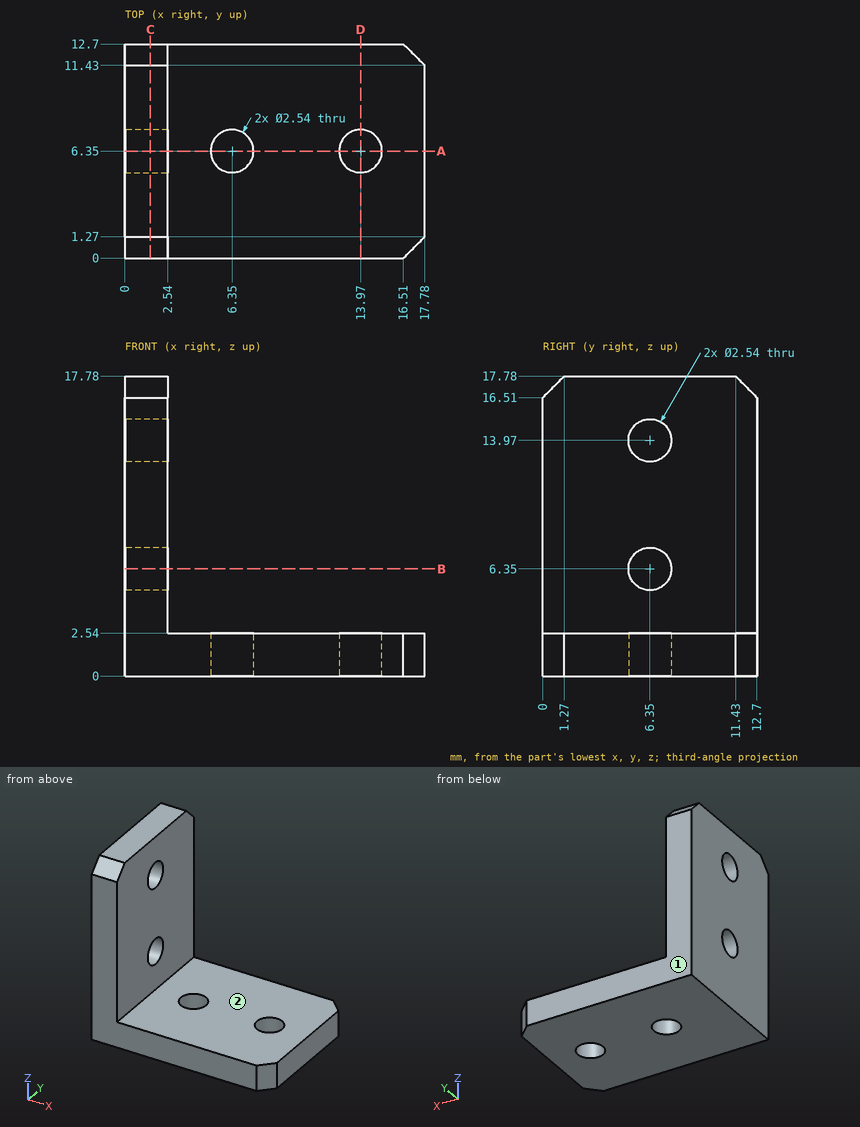
Source: three-view drawing plus pictorial views. Frame: mm from the lowest corner of the part. A direction names the side the tool comes from. Round coordinates to 2 decimals unless told otherwise and drop trailing zeros. Loops run counter-clockwise (first coordinate to the right, second up) from the corner with the lowest first, then second, coordinate; pieces in that order, holes last.
Q1. Section D-D, the plane x = 13.97. Return loops of the section in (y, z), plus the area to 3 significant figures.
Q2. Section A-A, the plane y = 6.35. Return loops of the section in (x, z), plus the area to 3 significant figures.
Q3. Section B-B, the plane z = 6.35. Return loops of the section in (x, y).
Q4. Ray query, line 1 (Y direction, x = 13.97, z = 1.9); line 2 (X direction, y = 11.5, z = 6.25). Return the intervals inside material, ascending.
Q5. Access query for the marked faces 1 and 2. Directions: +Z, -Z, +X, -X, +Y, -Y. A direction counts if a zero-diameter tool reaches every point of the face in a straight line with its end or side. Return the directions, or none.
Q6. Section C-C, the plane x = 1.5. Return loops of the section in (y, z).
Q7. First-contact query: P1, Ø1.5, axis at y = 4.5, z = 12.5, coming from the +X side; P2, Ø1, axis at x = 14, y = 8.5, coming from the +Z side. Flat tips, straight axial feed; report the tip coordinate or a pass-through.
Solutions:
1. outline: (0, 0) - (5.08, 0) - (5.08, 2.54) - (0, 2.54) - close; (7.62, 0) - (12.7, 0) - (12.7, 2.54) - (7.62, 2.54) - close
1. area: 25.8 mm2
2. outline: (0, 0) - (5.08, 0) - (5.08, 2.54) - (2.54, 2.54) - (2.54, 5.08) - (0, 5.08) - close; (0, 7.62) - (2.54, 7.62) - (2.54, 12.7) - (0, 12.7) - close; (0, 15.24) - (2.54, 15.24) - (2.54, 17.78) - (0, 17.78) - close; (7.62, 0) - (12.7, 0) - (12.7, 2.54) - (7.62, 2.54) - close; (15.24, 0) - (17.78, 0) - (17.78, 2.54) - (15.24, 2.54) - close
2. area: 58.1 mm2
3. outline: (0, 0) - (2.54, 0) - (2.54, 5.08) - (0, 5.08) - close; (0, 7.62) - (2.54, 7.62) - (2.54, 12.7) - (0, 12.7) - close
4. line 1: y = 0 to 5.08, 7.62 to 12.7
4. line 2: x = 0 to 2.54
5. face 1: +Z, -Z, +X, -X, +Y
5. face 2: +Z, +X, +Y, -Y
6. outline: (0, 0) - (12.7, 0) - (12.7, 16.51) - (11.43, 17.78) - (1.27, 17.78) - (0, 16.51) - close; hole circle Ø2.54 at (6.35, 6.35); hole circle Ø2.54 at (6.35, 13.97)
7. P1: stops at x = 2.54
7. P2: stops at z = 2.54
